For this review, take the finished solid that the model builds, in its own axes (mm). Face numbers are marked on the shaded views. A direction names the side the tool comes from. Coordinates: 2 decimals unless noted, no trailing zeros. Write each loop counter-clockwise with the first axis right and the second up, starting at its lowest first coordinate (ties: lowest second). Pieces come first, ordered by that corner, then holes. Notation, with made-up numbers: (83, -13) -> (108, -13) arc R12 ccw to (108, -3) -> close; hole circle Ø7 at (50, 3). An arc over 180 degrees is marked (long way). One line per item, written item: value. Start each with the question number.
1) Mouldability with a two-part tool opening along Z and no side actions: class the marked faces 4, 5 and 6 as released by +Z, released by -Z, zero draft, split by the parting line, or undercut.
2) Add section D-D (z = -8.5). State the section outline as (x, y) points.
3) Add section B-B (x = 0). State the section outline as (y, z) points, and give its area (3 significant figures).
4) Add section A-A (y = 55). State the section outline as (x, z) points.
5) For pin 1 Ø10.5 at (x, y) = (1, 35.5) entering from -Z; pin 2 Ø23 at (y, z) = (45, 0.5) entering from -X; pin 3 Ø1.5 at (x, y) = (7.5, 54) entering from +Z, all flat-tipped, find the tip position at first contact; note any pin that passes through.
6) For probe 1 along X at (y, z) = (49, 0); probe 2 along Z at (x, y) = (-7, 7.5); probe 3 along Y at (x, z) = (-8.5, -1.5), list the stretches that pass through material, from the lowest coordinate up. Write a range as from..to.
7) Machinability: for the marked faces 1, 2 and 3, which of the approach directions +Z, -Z, +X, -X, +Y, -Y give a long, thin tool a straight path to every point of the face, cutting with its end or side? Answer none if there is none.
8) Add section C-C (z = 0). State the section outline as (x, y) points.
from build123d import *

# Parameters (mm, degrees)
SKETCH1_R           = 26.5
BOSS_EXTRUDE1_DEPTH = 3
SKETCH10_W          = 27
SKETCH10_H          = 27
BOSS_EXTRUDE6_DEPTH = 90
SKETCH11_R          = 5.5
CUT_EXTRUDE3_DEPTH  = 90
SKETCH12_R          = 11.5
CUT_EXTRUDE4_DEPTH  = 6
FILLET2_R           = 3


with BuildPart() as part:
    # Sketch1 → Boss-Extrude1 (new body)
    with BuildSketch(Plane(origin=(0, 0, 0), x_dir=(1, 0, 0), z_dir=(0, 1, 0))):
        with Locations(Location((0, 0, 0), (0, 0, 270))):
            Circle(SKETCH1_R)
    extrude(amount=BOSS_EXTRUDE1_DEPTH)

    # Sketch10 → Boss-Extrude6 (add)
    with BuildSketch(Plane(origin=(0, 3, 0), x_dir=(1, 0, 0), z_dir=(0, 1, 0))):
        Rectangle(SKETCH10_W, SKETCH10_H)
    extrude(amount=BOSS_EXTRUDE6_DEPTH)

    # Sketch11 → Cut-Extrude3 (cut)
    with BuildSketch(Plane(origin=(0, 93, 0), x_dir=(1, 0, 0), z_dir=(0, 1, 0))):
        with Locations(Location((0, 0, 0), (0, 0, 270))):
            Circle(SKETCH11_R)
    extrude(amount=-CUT_EXTRUDE3_DEPTH, mode=Mode.SUBTRACT)

    # Sketch12 → Cut-Extrude4 (cut)
    with BuildSketch(Plane(origin=(0, 93, 0), x_dir=(1, 0, 0), z_dir=(0, 1, 0))):
        with Locations(Location((0, 0, 0), (0, 0, 270))):
            Circle(SKETCH12_R)
    extrude(amount=-CUT_EXTRUDE4_DEPTH, mode=Mode.SUBTRACT)

    # Fillet2
    fillet2_edges = [part.edges().sort_by_distance(p)[0] for p in [
        (13.5, 48, 13.5),
        (13.5, 48, -13.5),
        (-13.5, 48, -13.5),
        (-13.5, 48, 13.5),
    ]]
    fillet(fillet2_edges, radius=FILLET2_R)


solid = part.part
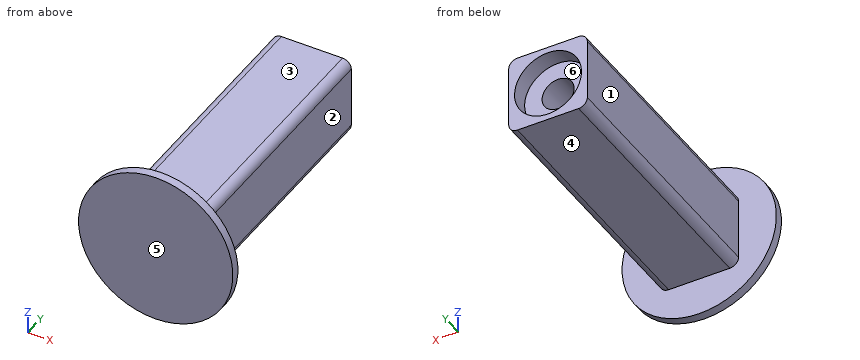
Numbers:
1. face 4: released by -Z
1. face 5: zero draft
1. face 6: undercut
2. outline: (-25.1, 0) -> (25.1, 0) -> (25.1, 3) -> (13.5, 3) -> (13.5, 93) -> (7.75, 93) -> (7.75, 87) -> (-7.75, 87) -> (-7.75, 93) -> (-13.5, 93) -> (-13.5, 3) -> (-25.1, 3) -> close
3. outline: (0, -26.5) -> (3, -26.5) -> (3, -13.5) -> (93, -13.5) -> (93, -11.5) -> (87, -11.5) -> (87, -5.5) -> (3, -5.5) -> (3, 5.5) -> (87, 5.5) -> (87, 11.5) -> (93, 11.5) -> (93, 13.5) -> (3, 13.5) -> (3, 26.5) -> (0, 26.5) -> close
3. area: 1,530 mm²
4. outline: (-13.5, -10.5) arc R3 ccw to (-10.5, -13.5) -> (10.5, -13.5) arc R3 ccw to (13.5, -10.5) -> (13.5, 10.5) arc R3 ccw to (10.5, 13.5) -> (-10.5, 13.5) arc R3 ccw to (-13.5, 10.5) -> close; hole circle Ø11 at (0, 0)
5. pin 1: z = -13.5
5. pin 2: x = -13.5
5. pin 3: z = 13.5
6. probe 1: -13.5..-5.5, 5.5..13.5
6. probe 2: -13.5..13.5
6. probe 3: 0..87
7. face 1: +Z, -Z, -X, +Y
7. face 2: +Z, -Z, +X, +Y
7. face 3: +Z, +X, -X, +Y
8. outline: (-26.5, 0) -> (26.5, 0) -> (26.5, 3) -> (13.5, 3) -> (13.5, 93) -> (11.5, 93) -> (11.5, 87) -> (5.5, 87) -> (5.5, 3) -> (-5.5, 3) -> (-5.5, 87) -> (-11.5, 87) -> (-11.5, 93) -> (-13.5, 93) -> (-13.5, 3) -> (-26.5, 3) -> close
